```python
from build123d import *

# Parameters (mm, degrees)
SKETCH4_W               = 12
SKETCH4_H               = 13.7
BOSS_EXTRUDE2_DEPTH     = 6.5
CUT_EXTRUDE1_DEPTH      = 3
CUT_EXTRUDE2_DEPTH      = 12.188051662
CUT_EXTRUDE2_DEPTH_BACK = 12.188051662
SKETCH5_R               = 1.6


with BuildPart() as part:
    # Sketch4 → Boss-Extrude2 (new body)
    with BuildSketch(Plane(origin=(0, 0, 0), x_dir=(1, 0, 0), z_dir=(0, 1, 0))):
        Rectangle(SKETCH4_W, SKETCH4_H)
    extrude(amount=BOSS_EXTRUDE2_DEPTH)

    # Sketch3 → Cut-Extrude1 (cut)
    with BuildSketch(Plane.XZ):
        Polygon((1.638566399, -2.920348179), (3.348378911, -0.041133962), (1.709812512, 2.879214217), (-1.638566399, 2.920348179), (-3.348378911, 0.041133962), (-1.709812512, -2.879214217), align=None)
    extrude(amount=-CUT_EXTRUDE1_DEPTH, mode=Mode.SUBTRACT)

    # Sketch5 → Cut-Extrude2 (cut, two sides: drawn at the far end of the back side and taken through both)
    with BuildSketch(Plane.XZ.offset(-CUT_EXTRUDE2_DEPTH_BACK)):
        with Locations(Location((0, 0, 0), (0, 0, 270))):
            Circle(SKETCH5_R)
    extrude(amount=CUT_EXTRUDE2_DEPTH + CUT_EXTRUDE2_DEPTH_BACK, mode=Mode.SUBTRACT)


solid = part.part
```
CAD build for the part. Positions are in the model's coordinates, mm. A direction names the side the tool comes from. Round coordinates to 2 decimals unless told otherwise and drop trailing zeros. Write each loop counter-clockwise with the first axis right and the second up, starting at its lowest first coordinate (ties: lowest second). Pieces come first, ordered by that corner, then holes. Notation, with made-up numbers: (-31, 1.25) - (14, 1.25) arc R26 ccw to (14, 31.25) - close; hole circle Ø3 at (0.25, 59.25). An arc over 180 degrees is marked (long way). Return JSON: item names as keys, results as strings. Group by question number.
Item 1: Band-saw the part on D-D on x = -1. List the corners of the cut face in (y, z).
Item 2: Band-saw the part on A-A on y = 1. List the corners of the cut face in (x, z).
Item 3: Mould opens along Z. For faces 3 (the face through (0, 3, -6.85)), 4 (the face through (2.48, 1.48, -1.5)), 5 (the face through (-2.48, 1.48, 1.5)), 6 (the face through (0, 3, 6.85)) say: +Z half, -Z half, draft (parallel to the pull), parting line (faces both ways), or undercut.
Item 4: Band-saw the part on B-B on x = 1.25. List the corners of the cut face in (y, z), plus the area to 3 significant figures.
Item 5: Band-saw the part on C-C on x = -2.75. List the corners of the cut face in (y, z).
Item 6: Probe probe 1 along Z at (x, y) = (0, 5.4); probe 2 along X at (y, z) = (4, 0); probe 3 along Y at (x, z) = (2.5, -0.5). List the from-to ranges inside material, lowest first.
Item 7: Flat gauge pin, fed straight in: pin 1 Ø1.8 at (x, z) = (-1.5, 0) entering from -Y. Where does the tip first touch, or does it go through?
Item 8: 3-axis set-ups, long thin cutter, end or side, ignore diameter. For faces 1 (the face through (-2, 3, 1)), 2 (the face through (-6, 3, 0)): which of +Z, -Z, +X, -X, +Y, -Y reach the whole face in a straight line?
Resolved:
{
 "1": {"outline": "(0, -6.85) - (6.5, -6.85) - (6.5, -1.25) - (3, -1.25) - (3, -2.89) - (0, -2.89) - close; (0, 2.91) - (3, 2.91) - (3, 1.25) - (6.5, 1.25) - (6.5, 6.85) - (0, 6.85) - close"},
 "2": {"outline": "(-6, -6.85) - (6, -6.85) - (6, 6.85) - (-6, 6.85) - close; hole (-3.35, 0.04) - (-1.71, -2.88) - (1.64, -2.92) - (3.35, -0.04) - (1.71, 2.88) - (-1.64, 2.92) - close"},
 "3": {"face 3": "-Z half", "face 4": "undercut", "face 5": "undercut", "face 6": "+Z half"},
 "4": {"outline": "(0, -6.85) - (6.5, -6.85) - (6.5, -1) - (3, -1) - (3, -2.92) - (0, -2.92) - close; (0, 2.88) - (3, 2.88) - (3, 1) - (6.5, 1) - (6.5, 6.85) - (0, 6.85) - close", "area": "64.7 mm²"},
 "5": {"outline": "(0, -6.85) - (6.5, -6.85) - (6.5, 6.85) - (0, 6.85) - (0, 1.05) - (3, 1.05) - (3, -1.03) - (0, -1.03) - close"},
 "6": {"probe 1": "z = -6.85 to -1.6, 1.6 to 6.85", "probe 2": "x = -6 to -1.6, 1.6 to 6", "probe 3": "y = 3 to 6.5"},
 "7": {"pin 1": "stops at y = 3"},
 "8": {"face 1": "-Y", "face 2": "+Z, -Z, -X, +Y, -Y"}
}
